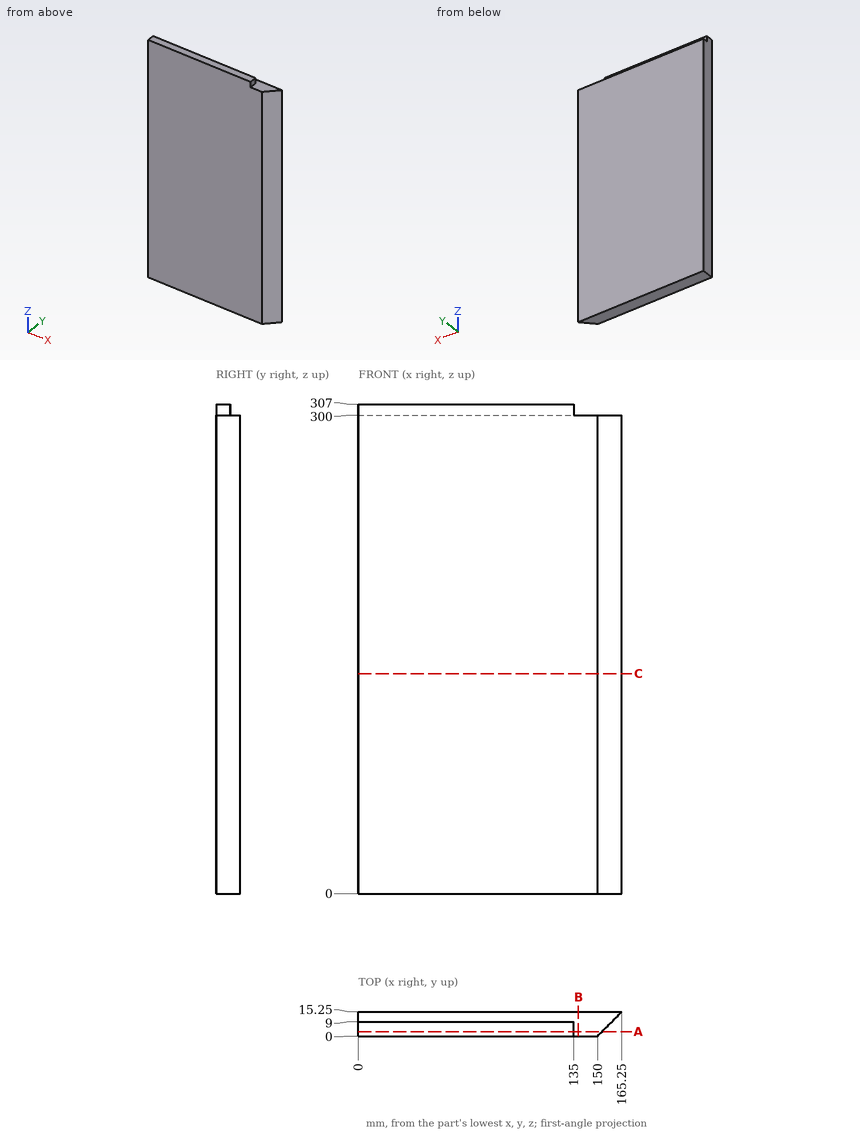
The drawing under review shows one solid part. Ordinate dimensions are in mm from its lowest x, y, z. Coordinates: 2 decimals unless noted, no trailing zeros. Write each loop counter-clockwise with the first axis right and the second up, starting at its lowest first coordinate (ties: lowest second). Pieces come first, ordered by that corner, then holes. Notation, with made-up numbers: (75, 50.25) -> (80, 50.25) arc R11 ccw to (80, 54.25) -> close; hole circle Ø3 at (9.5, 10). An arc over 180 degrees is marked (long way). One line per item, written item: value. Start each with the question number.
Q1. Add section C-C, the plane z = 138. Give the boundary of the cut face in (x, y), then the cut area to 3 significant figures.
Q2. Add section B-B, the plane x = 138. Give the boundary of the cut face in (y, z).
Q3. Add section A-A, the plane y = 2.75. Give the boundary of the cut face in (x, z).
Q4. To check wall thickness, follow probe 1 along Z at (x, y) = (145, 7.5); probe 2 along X at (y, z) = (5, 291); probe 3 along X at (y, z) = (1.25, 197). State the ranges of each line that lie inside material, in increasing order.
Q5. Clearance check with flat-ended pins moving along their axes: P1, Ø1.5, axis at y = 4.5, z = 239, coming from the -X side; P2, Ø8, axis at y = 9.5, z = 168, coming from the +X side; P3, Ø5.5, axis at y = 6, z = 302.5, coming from the +X side; P4, Ø2, axis at y = 5.5, z = 276, coming from the +X side. State where each tip first meets the part, or that it passes through.
Response:
1. outline: (0, 0) -> (150, 0) -> (165.25, 15.25) -> (0, 15.25) -> close
1. area: 2,400 mm²
2. outline: (0, 0) -> (15.25, 0) -> (15.25, 300) -> (0, 300) -> close
3. outline: (0, 0) -> (152.75, 0) -> (152.75, 300) -> (135, 300) -> (135, 307) -> (0, 307) -> close
4. probe 1: 0 to 300
4. probe 2: 0 to 155
4. probe 3: 0 to 151.25
5. P1: x = 0
5. P2: x = 163.5
5. P3: x = 157.15
5. P4: x = 156.5
